Geometry check sheet. Reference: the model listing, model coordinates, mm. Face numbers are marked on the shaded views. A direction names the side the tool comes from. Give positions to 0.01 mm unless a question says otherwise; leave off trailing zeros. Write each loop counter-clockwise with the first axis right and the second up, starting at its lowest first coordinate (ties: lowest second). Pieces come first, ordered by that corner, then holes. Notation, with made-up numbers: (24.5, 10.25) - (64.5, 10.25) arc R16 ccw to (64.5, 29.25) - close; hole circle Ø3 at (-9, -14.75). An arc over 180 degrees is marked (long way). Write item = value, one per line. Start each with the question number.
(1) Section check D-D, the plane x = 36. Enter the section's corners in (y, z).
(2) Thickness scan on L1, parallel to X at y = -6.5, z = 11.25; L2, parallel to X at y = -10.5, z = 4.5; L3, parallel to X at y = -8, z = 9. Record the ranges inside material, lowest first.
(3) Section check B-B, the plane y = -16.5. Enter the section's corners in (x, z).
(4) Draft check along X on the marked faces 5, 6 and 7. Enter one of: pulls with the +X half, pulls with the -X half, needs draft (parallel to the pull), parting line crosses it, or undercut.
(5) Depth check by flat-ended pin: pin 1 Ø2 at (x, z) = (69, 8.5) entering from -Y; pin 2 Ø13.5 at (x, y) = (10.67, -10.67) entering from -Z; pin 3 Ø5.5 at (x, y) = (46.01, -7.7) entering from +Z; pin 4 Ø4.5 at (x, y) = (66.69, -10.67) entering from -Z. Enter the tip coordinate at first touch or a pass-through.
(6) Section check A-A, the plane z = 4. Give the number of separate pieces and of enclosed holes in the cut face, plus the area to 3 significant figures.
(7) Access from +Z, -Z, +X, -X, +Y, -Y to the whole of each face (thin tool, end or side, straight path). Record for the marked faces 1, 2, 3 and 4.
(8) Section check C-C, the plane x = 16.5. Enter the section's corners in (y, z), plus the area to 3 significant figures.
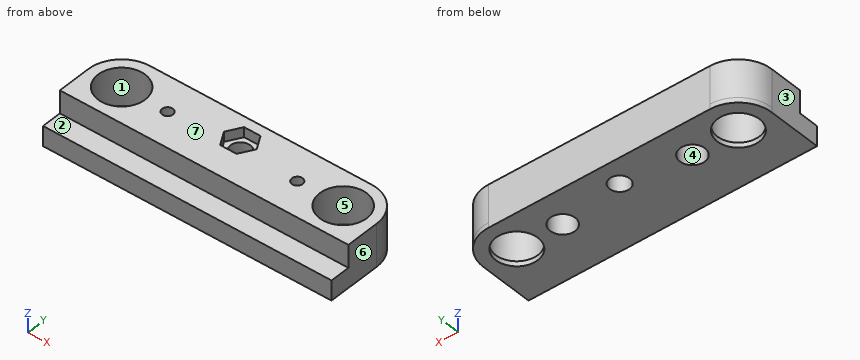
```python
from build123d import *

# Parameters (mm, degrees)
F0_W      = 92.0124906
F0_H      = 27.6999954
F0_R      = 6.7062477
F1_DEPTH  = 1.5875
F2_R      = 10.6749977
F3_R      = 7.5
F4_DEPTH  = 12
F5_DEPTH  = 4.7625
F6_R      = 1.7272
F6_R_2    = 3.175
F7_DEPTH  = 13.5875
F8_R      = 3.96875
F9_DEPTH  = 7.2375014
F11_DEPTH = 3.175


with BuildPart() as f1:
    # F0 (on Top) → F1 (new body)
    with BuildSketch(Plane.XY):
        with Locations((46.0062453, -13.8499977)):
            Rectangle(F0_W, F0_H)
        with Locations((10.6749977, -10.6749977)):
            Circle(F0_R, mode=Mode.SUBTRACT)
        with Locations((81.3374929, -10.6749977)):
            Circle(F0_R, mode=Mode.SUBTRACT)
    extrude(amount=F1_DEPTH)

    # F2
    f2_edges = [f1.edges().sort_by_distance(p)[0] for p in [
        (0, 0, 0.79375),
        (92.012491, 0, 0.79375),
    ]]
    fillet(f2_edges, radius=F2_R)

    # F3 (on face) → F4 (join)
    with BuildSketch(Plane.XY.offset(1.5875)):
        with BuildLine():
            Line((0, -10.6749977), (0, -21.3499954))
            Line((0, -21.3499954), (92.0124906, -21.3499954))
            Line((92.0124906, -21.3499954), (92.0124906, -10.6749977))
            ThreePointArc((92.0124906, -10.6749977), (88.8858561628, -3.1266344372), (81.3374929, 0))
            Line((81.3374929, 0), (10.6749977, 0))
            ThreePointArc((10.6749977, 0), (3.1266344372, -3.1266344372), (0, -10.6749977))
        make_face()
        with Locations((10.6749977, -10.6749977)):
            Circle(F3_R, mode=Mode.SUBTRACT)
        with Locations((81.3374929, -10.6749977)):
            Circle(F3_R, mode=Mode.SUBTRACT)
    extrude(amount=F4_DEPTH)

    # F5 (add): a face of the model
    f5_faces = [f1.faces().sort_by_distance(p)[0] for p in [
        (46.0062453, -24.5249954, 1.5875),
    ]]
    extrude(f5_faces, amount=F5_DEPTH)

    # F6 (on face) → F7 (cut, through all)
    with BuildSketch(Plane.XY.offset(13.5875)):
        with Locations((25.3187477, -10.6749977)):
            Circle(F6_R)
        with Locations((66.6937429, -10.6749977)):
            Circle(F6_R)
        with Locations((46.0062453, -7.6956539)):
            Circle(F6_R_2)
    extrude(amount=-F7_DEPTH, mode=Mode.SUBTRACT)

    # F8 (on face) → F9 (cut)
    with BuildSketch(Plane(origin=(0, 0, 0), x_dir=(1, 0, 0), z_dir=(0, 0, -1))):
        with Locations((66.6937429, 10.6749977)):
            Circle(F8_R)
        with Locations((25.3187477, 10.6749977)):
            Circle(F8_R)
    extrude(amount=-F9_DEPTH, mode=Mode.SUBTRACT)

    # F10 (on face) → F11 (cut)
    with BuildSketch(Plane.XY.offset(13.5875)):
        Polygon((48.6162460461, -3.175), (43.3962445539, -3.175), (40.7862438078, -7.6956539), (43.3962445539, -12.2163078), (48.6162460461, -12.2163078), (51.2262467922, -7.6956539), align=None)
    extrude(amount=-F11_DEPTH, mode=Mode.SUBTRACT)


solid = f1.part
```
Model answer:
q1.outline = (-27.7, 0) - (0, 0) - (0, 13.59) - (-21.35, 13.59) - (-21.35, 6.35) - (-27.7, 6.35) - close
q2.L1 = 0.85 to 4.44, 16.91 to 41.48, 50.54 to 75.11, 87.57 to 91.16
q2.L2 = 0 to 3.18, 18.17 to 21.35, 29.28 to 44.52, 47.49 to 62.73, 70.66 to 73.84, 88.84 to 92.01
q2.L3 = 0.34 to 3.67, 17.68 to 42.85, 49.17 to 74.33, 88.34 to 91.67
q3.outline = (0, 0) - (7.35, 0) - (7.35, 1.59) - (5.95, 1.59) - (5.95, 13.59) - (0, 13.59) - close; (14, 0) - (78.01, 0) - (78.01, 1.59) - (76.61, 1.59) - (76.61, 13.59) - (15.4, 13.59) - (15.4, 1.59) - (14, 1.59) - close; (84.66, 0) - (92.01, 0) - (92.01, 13.59) - (86.06, 13.59) - (86.06, 1.59) - (84.66, 1.59) - close
q4.face_5 = undercut
q4.face_6 = pulls with the +X half
q4.face_7 = needs draft
q5.pin_1 = -21.35
q5.pin_2 = 0
q5.pin_3 = through
q5.pin_4 = 7.24
q6.separate_pieces = 1
q6.enclosed_holes = 5
q6.area = 2,020 mm²
q7.face_1 = +Z
q7.face_2 = +Z, +X, -X, -Y
q7.face_3 = +Z, -Z, -X, +Y, -Y
q7.face_4 = -Z
q8.outline = (-27.7, 0) - (-14, 0) - (-14, 1.59) - (-15.4, 1.59) - (-15.4, 13.59) - (-21.35, 13.59) - (-21.35, 6.35) - (-27.7, 6.35) - close; (-7.35, 0) - (0, 0) - (0, 13.59) - (-5.95, 13.59) - (-5.95, 1.59) - (-7.35, 1.59) - close
q8.area = 206 mm²
